```python
from build123d import *

# Parameters (mm, degrees)
BOSS_EXTRUDE1_DEPTH = 563.88
SHELL1_T            = -6.35
SKETCH2_W           = 563.88
SKETCH2_H           = 25.4
BOSS_EXTRUDE2_DEPTH = 7.62


with BuildPart() as part:
    # Sketch1 → Boss-Extrude1 (new body)
    with BuildSketch(Plane.XY):
        with BuildLine():
            Line((0, 0), (0, 133.572018751))
            ThreePointArc((0, 133.572018751), (181.379040374, 111.770166328), (352.425, 47.606650594))
            Line((352.425, 47.606650594), (326.303398408, -50.577981249))
            Line((326.303398408, -50.577981249), (0, 0))
        make_face()
    extrude(amount=BOSS_EXTRUDE1_DEPTH)

    # Shell1
    shell1_openings = [part.faces().sort_by_distance(p)[0] for p in [
        (181.379040374, 111.770166328, 281.94),
    ]]
    offset(amount=SHELL1_T, openings=shell1_openings, kind=Kind.INTERSECTION)

    # Sketch2 → Boss-Extrude2 (add)
    with BuildSketch(Plane.ZY):
        with Locations((281.94, 82.772018751)):
            Rectangle(SKETCH2_W, SKETCH2_H)
    extrude(amount=BOSS_EXTRUDE2_DEPTH)


solid = part.part
```
Work out the finished part from the listing and answer in its coordinate system (mm). A direction names the side the tool comes from. Round coordinates to 2 decimals unless told otherwise and drop trailing zeros. Write each loop counter-clockwise with the first axis right and the second up, starting at its lowest first coordinate (ties: lowest second). Pieces come first, ordered by that corner, then holes.
1) A cutting plane is placed at C-C on x = 155. Determine the outline of the cut face in (y, z).
2) A cutting plane is placed at B-B on z = 231.5. Determine the outline of the cut face in (x, y) (3 decimals).
3) Determine the mould class of faces 1 (the face through (175, 43, 563.88)), 2 (the face through (179, 46, 6.35)), 3 (the face through (-7.62, 83, 278)) for opening direction X: pulls with the +X half, pulls with the -X half, needs draft (parallel to the pull), parting line crosses it, or undercut.
4) Which of the six approach directions +Z, -Z, +X, -X, +Y, -Y give full straight-line access (tool end or side, diameter ignored) to faces 4 (the face through (0, 114, 278)), 5 (the face through (0, 35, 278)), 6 (the face through (334.314, 4.231, 278.082))?
5) A cutting plane is placed at A-A on y = 21.5. Determine the outline of the cut face in (x, z), and give its area (3 significant figures).
6) A cutting plane is placed at D-D on y = 86. Determine the outline of the cut face in (x, z).
7) Flat-ended cylindrical pins translate along their axes: P1, Ø6, axis at x = 196, z = 466, coming from the -Y side; P2, Ø1, axis at y = 37.5, z = 269, coming from the -X side; P3, Ø1.5, axis at x = 78, z = 476.5, coming from the -Y side. Find the tip coordinate at first contact, or state that the pin passes through.
8) Consider probe 1 along Z at (x, y) = (16, 50); probe 2 along X at (y, z) = (6.5, 62.5). Determine where each line is inside the solid, lowest interval first.
Entries:
1. outline: (-24.03, 0) - (117.71, 0) - (117.71, 6.35) - (-17.6, 6.35) - (-17.6, 557.53) - (117.71, 557.53) - (117.71, 563.88) - (-24.03, 563.88) - close
2. outline: (-7.62, 70.072) - (0, 70.072) - (0, 0) - (326.303, -50.578) - (352.425, 47.607) arc R765.386 ccw to (346.644, 50.574) - (321.635, -43.428) - (6.35, 5.442) - (6.35, 133.546) arc R765.386 ccw to (0, 133.572) - (0, 95.472) - (-7.62, 95.472) - close
3. face 1: needs draft
3. face 2: undercut
3. face 3: pulls with the -X half
4. face 4: +Z, -Z, -X, +Y
4. face 5: +Z, -Z, -X, -Y
4. face 6: +Y
5. outline: (0, 0) - (345.48, 0) - (345.48, 563.88) - (0, 563.88) - close; hole (6.35, 6.35) - (338.91, 6.35) - (338.91, 557.53) - (6.35, 557.53) - close
5. area: 11,500 mm2
6. outline: (-7.62, 0) - (265.63, 0) - (265.63, 6.35) - (6.35, 6.35) - (6.35, 557.53) - (265.63, 557.53) - (265.63, 563.88) - (-7.62, 563.88) - close
7. P1: stops at y = -30.85
7. P2: stops at x = 0
7. P3: stops at y = -12.21
8. probe 1: z = 0 to 6.35, 557.53 to 563.88
8. probe 2: x = 0 to 6.35, 334.92 to 341.49
